```python
from build123d import *

# Parameters (mm, degrees)
F0_W     = 40
F0_H     = 40
F1_DEPTH = 10
F2_W     = 10
F2_H     = 40
F3_DEPTH = 50
F4_W     = 10
F4_H     = 40
F5_DEPTH = 50
F6_R     = 7
F7_DEPTH = 96.2
F8_SIZE  = 5


with BuildPart() as f1:
    # F0 (on Top) → F1 (new body)
    with BuildSketch(Plane.XY):
        Rectangle(F0_W, F0_H)
    extrude(amount=F1_DEPTH)

    # F2 (on face) → F3 (join)
    with BuildSketch(Plane.XY.offset(10)):
        with Locations((-15, 0)):
            Rectangle(F2_W, F2_H)
    extrude(amount=F3_DEPTH)

    # F4 (on face) → F5 (join)
    with BuildSketch(Plane.XY.offset(10)):
        with Locations((15, 0)):
            Rectangle(F4_W, F4_H)
    extrude(amount=F5_DEPTH)

    # F6 (on face) → F7 (cut)
    with BuildSketch(Plane.YZ.offset(20)):
        with Locations((0, 40)):
            Circle(F6_R)
    extrude(amount=-F7_DEPTH, mode=Mode.SUBTRACT)

    # F8
    f8_edges = [f1.edges().sort_by_distance(p)[0] for p in [
        (-15, -20, 60),
        (15, -20, 60),
        (15, 20, 60),
        (-15, 20, 60),
    ]]
    chamfer(f8_edges, length=F8_SIZE)


solid = f1.part
```
Source: CAD feature listing. Evaluate the final solid. Frame: model axes, mm. A direction names the side the tool comes from. Coordinates: 2 decimals unless noted, no trailing zeros. Write each loop counter-clockwise with the first axis right and the second up, starting at its lowest first coordinate (ties: lowest second). Pieces come first, ordered by that corner, then holes. Notation, with made-up numbers: (49, -7) - (94, -7) arc R14 cw to (94, 6) - close; hole circle Ø6 at (45.5, 28.5). An arc over 180 degrees is marked (long way). Answer as a JSON object with one key per item and string values.
Q1. Draft query along Z for faces 1 (the flat face through (-10, -4.7, 34.6)), 2 (the flat face through (-15, -17, 58)), 3 (the cylindrical face through (-14.93, -0.91, 46.94)). Return one class per face: released by +Z, released by -Z, zero draft, split by the parting line, or undercut.
Ans:
{"face 1": "zero draft", "face 2": "released by +Z", "face 3": "undercut"}
Q2. Set-up query: faces 4 (the flat face through (-14, -20, 21)), 5 (the flat face through (0, 0, 10)). Return all of +Z, -Z, +X, -X, +Y, -Y with unobstructed straight access to the full face (end or side cutting, diameter ignored); none if empty.
Ans:
{"face 4": "+Z, -Z, +X, -X, -Y", "face 5": "+Z, +Y, -Y"}
Q3. Section query C-C, the plane y = 0. Output: boundary loops of the cut face in (x, z).
Ans:
{"outline": "(-20, 0) - (20, 0) - (20, 33) - (10, 33) - (10, 10) - (-10, 10) - (-10, 33) - (-20, 33) - close; (-20, 47) - (-10, 47) - (-10, 60) - (-20, 60) - close; (10, 47) - (20, 47) - (20, 60) - (10, 60) - close"}
Q4. Section query D-D, the plane z = 40. Output: boundary loops of the cut face in (x, y).
Ans:
{"outline": "(-20, -20) - (-10, -20) - (-10, -7) - (-20, -7) - close; (-20, 7) - (-10, 7) - (-10, 20) - (-20, 20) - close; (10, -20) - (20, -20) - (20, -7) - (10, -7) - close; (10, 7) - (20, 7) - (20, 20) - (10, 20) - close"}
Q5. Material intervals for line 1 (X direction, y = 3, z = 20); line 2 (Z direction, x = 17, y = 0); line 3 (Z direction, x = 16.5, y = 4), sorted ascending. Write a range as [from, to].
Ans:
{"line 1": "x = [-20, -10], [10, 20]", "line 2": "z = [0, 33], [47, 60]", "line 3": "z = [0, 34.26], [45.74, 60]"}
Q6. First-contact query: pin 1 Ø6 at (x, y) = (8.5, -5) entering from -Z; pin 2 Ø12.5 at (y, z) = (0, 40) entering from -X. Flat tips, straight axial feed; report the tip coordinate or a pass-through.
Ans:
{"pin 1": "stops at z = 0", "pin 2": "passes through"}
Q7. Section query B-B, the plane z = 15. Output: boundary loops of the cut face in (x, y).
Ans:
{"outline": "(-20, -20) - (-10, -20) - (-10, 20) - (-20, 20) - close; (10, -20) - (20, -20) - (20, 20) - (10, 20) - close"}
Q8. Section query A-A, the plane x = -16.5. Output: boundary loops of the cut face in (y, z).
Ans:
{"outline": "(-20, 0) - (20, 0) - (20, 55) - (15, 60) - (-15, 60) - (-20, 55) - close; hole circle Ø14 at (0, 40)"}
